Source: CAD feature listing. Evaluate the final solid. Frame: model axes, mm. A direction names the side the tool comes from. Round coordinates to 2 decimals unless told otherwise and drop trailing zeros. Loops run counter-clockwise (first coordinate to the right, second up) from the corner with the lowest first, then second, coordinate; pieces in that order, holes last. Notation, with made-up numbers: (26, -5) -> (32, -5) arc R24 ccw to (32, 33) -> close; hole circle Ø3 at (-34.5, 10). An arc over 180 degrees is marked (long way). Write item = value, one per line.
from build123d import *

# Parameters (mm, degrees)
F1_DEPTH = 556
F3_DEPTH = 75.001
F5_DEPTH = 75.001
F7_W     = 75
F7_H     = 75
F8_DEPTH = 556.001


with BuildPart() as f1:
    # F0 (on Top) → F1 (new body)
    with BuildSketch(Plane.XY):
        Polygon((0, 75), (0, 0), (75, 0), (75, 6), (6, 6), (6, 75), align=None)
    extrude(amount=F1_DEPTH)

    # F2 (on Front) → F3 (cut, through all)
    with BuildSketch(Plane.XZ):
        Polygon((0, 75), (0, 0), (75, 0), align=None)
    extrude(amount=-F3_DEPTH, mode=Mode.SUBTRACT)

    # F4 (on Front) → F5 (cut, through all)
    with BuildSketch(Plane.XZ):
        Polygon((0, 481), (75, 556), (0, 556), align=None)
    extrude(amount=-F5_DEPTH, mode=Mode.SUBTRACT)

    # F6: F1 across plane


with BuildPart() as f1_1:
    add(f1.part)
    add(f1.part.mirror(Plane.XZ))

    # F7 (on Top) → F8 (cut, through all)
    with BuildSketch(Plane.XY):
        with Locations((37.5, 37.5)):
            Rectangle(F7_W, F7_H)
    extrude(amount=F8_DEPTH, mode=Mode.SUBTRACT)


solid = f1_1.part
1. Section query C-C (z = 147). Return the cut outline in (x, y), then the cut area to 3 significant figures.
Evaluation:
outline = (0, -75) -> (6, -75) -> (6, -6) -> (75, -6) -> (75, 0) -> (0, 0) -> close
area = 864 mm²
2. Contact query for flat-ended pins moving along their axis: pin 1 Ø1.5 at (x, z) = (40, 291.5) entering from -Y; pin 2 Ø10 at (x, y) = (62, -8.5) entering from +Z; pin 3 Ø2 at (y, z) = (-61, 424) entering from +X; pin 4 Ø2 at (x, z) = (62, 158.5) entering from +Y. Output: stop coordinate, or through.
Evaluation:
pin_1 = -6
pin_2 = 547.33
pin_3 = 6
pin_4 = 0
3. Section query B-B (y = -19). Return the cut outline in (x, z).
Evaluation:
outline = (0, 75) -> (6, 69) -> (6, 487) -> (0, 481) -> close
4. Section query A-A (x = 63.5). Return the cut outline in (y, z).
Evaluation:
outline = (-6, 11.5) -> (0, 11.5) -> (0, 544.5) -> (-6, 544.5) -> close
5. Line query: probe 1 along Y at (x, z) = (34, 339); probe 2 along X at (y, z) = (-65.5, 129); probe 3 along Z at (x, y) = (5, -70). Output: solid intervals per line, ascending. Write a range as from..to.
Evaluation:
probe_1 = -6..0
probe_2 = 0..6
probe_3 = 70..486
6. Set-up query: faces 1 (the face through (37, 0, 274)), 2 (the face through (6, -40, 275)). Return all of +Z, -Z, +X, -X, +Y, -Y with unobstructed straight access to the full face (end or side cutting, diameter ignored); none if empty.
Evaluation:
face_1 = +Z, -Z, +X, -X, +Y
face_2 = +Z, -Z, +X, -Y
